```python
from build123d import *

# Parameters (mm, degrees)
F0_R     = 69.85
F1_DEPTH = 76.2
F2_DEPTH = 50.8
F3_DEPTH = 63.5
F4_DEPTH = 25.4


with BuildPart() as f1:
    # F0 (on Top) → F1 (new body)
    with BuildSketch(Plane.XY):
        Circle(F0_R)
        with BuildLine():
            ThreePointArc((33.3375, 57.7422437973), (52.8968339639, 40.5891682792), (64.4031044678, 17.2567598322))
            ThreePointArc((64.4031044678, 17.2567598322), (66.1045861321, 8.7028338663), (66.675, 0))
            ThreePointArc((66.675, 0), (66.1045861321, -8.7028338663), (64.4031044678, -17.2567598322))
            ThreePointArc((64.4031044678, -17.2567598322), (40.5891682792, -52.8968339639), (0, -66.675))
            ThreePointArc((0, -66.675), (-17.2567598322, -64.4031044678), (-33.3375, -57.7422437973))
            ThreePointArc((-33.3375, -57.7422437973), (-52.8968339639, -40.5891682792), (-64.4031044678, -17.2567598322))
            ThreePointArc((-64.4031044678, -17.2567598322), (-66.675, 0), (-64.4031044678, 17.2567598322))
            ThreePointArc((-64.4031044678, 17.2567598322), (-40.5891682792, 52.8968339639), (0, 66.675))
            ThreePointArc((0, 66.675), (17.2567598322, 64.4031044678), (33.3375, 57.7422437973))
        make_face(mode=Mode.SUBTRACT)
        with BuildLine():
            Line((-33.3375, -57.7422437973), (-31.75, -54.9926131403))
            ThreePointArc((-31.75, -54.9926131403), (-50.3779371085, -38.6563507421), (-61.3362899694, -16.435009364))
            Line((-61.3362899694, -16.435009364), (-64.4031044678, -17.2567598322))
            ThreePointArc((-64.4031044678, -17.2567598322), (-52.8968339639, -40.5891682792), (-33.3375, -57.7422437973))
        make_face()
        with BuildLine():
            ThreePointArc((-61.3362899694, 16.435009364), (-38.6563507421, 50.3779371085), (0, 63.5))
            Line((0, 63.5), (0, 66.675))
            ThreePointArc((0, 66.675), (-40.5891682792, 52.8968339639), (-64.4031044678, 17.2567598322))
            Line((-64.4031044678, 17.2567598322), (-61.3362899694, 16.435009364))
        make_face()
        with BuildLine():
            ThreePointArc((-61.3362899694, -16.435009364), (-63.5, 0), (-61.3362899694, 16.435009364))
            Line((-61.3362899694, 16.435009364), (-64.4031044678, 17.2567598322))
            ThreePointArc((-64.4031044678, 17.2567598322), (-66.675, 0), (-64.4031044678, -17.2567598322))
            Line((-64.4031044678, -17.2567598322), (-61.3362899694, -16.435009364))
        make_face()
        with BuildLine():
            ThreePointArc((61.3362899694, 16.435009364), (62.9567486972, 8.288413206), (63.5, 0))
            ThreePointArc((63.5, 0), (62.9567486972, -8.288413206), (61.3362899694, -16.435009364))
            Line((61.3362899694, -16.435009364), (64.4031044678, -17.2567598322))
            ThreePointArc((64.4031044678, -17.2567598322), (66.1045861321, -8.7028338663), (66.675, 0))
            ThreePointArc((66.675, 0), (66.1045861321, 8.7028338663), (64.4031044678, 17.2567598322))
            Line((64.4031044678, 17.2567598322), (61.3362899694, 16.435009364))
        make_face()
        with BuildLine():
            ThreePointArc((31.75, 54.9926131403), (50.3779371085, 38.6563507421), (61.3362899694, 16.435009364))
            Line((61.3362899694, 16.435009364), (64.4031044678, 17.2567598322))
            ThreePointArc((64.4031044678, 17.2567598322), (52.8968339639, 40.5891682792), (33.3375, 57.7422437973))
            Line((33.3375, 57.7422437973), (31.75, 54.9926131403))
        make_face()
        with BuildLine():
            Line((64.4031044678, -17.2567598322), (61.3362899694, -16.435009364))
            ThreePointArc((61.3362899694, -16.435009364), (38.6563507421, -50.3779371085), (0, -63.5))
            Line((0, -63.5), (0, -66.675))
            ThreePointArc((0, -66.675), (40.5891682792, -52.8968339639), (64.4031044678, -17.2567598322))
        make_face()
        with BuildLine():
            Line((0, -66.675), (0, -63.5))
            ThreePointArc((0, -63.5), (-16.435009364, -61.3362899694), (-31.75, -54.9926131403))
            Line((-31.75, -54.9926131403), (-33.3375, -57.7422437973))
            ThreePointArc((-33.3375, -57.7422437973), (-17.2567598322, -64.4031044678), (0, -66.675))
        make_face()
        with BuildLine():
            ThreePointArc((0, 63.5), (16.435009364, 61.3362899694), (31.75, 54.9926131403))
            Line((31.75, 54.9926131403), (33.3375, 57.7422437973))
            ThreePointArc((33.3375, 57.7422437973), (17.2567598322, 64.4031044678), (0, 66.675))
            Line((0, 66.675), (0, 63.5))
        make_face()
    extrude(amount=F1_DEPTH)

    # F0 (on Top) → F2 (cut)
    with BuildSketch(Plane.XY):
        with BuildLine():
            ThreePointArc((-61.3362899694, -16.435009364), (-63.5, 0), (-61.3362899694, 16.435009364))
            Line((-61.3362899694, 16.435009364), (-64.4031044678, 17.2567598322))
            ThreePointArc((-64.4031044678, 17.2567598322), (-66.675, 0), (-64.4031044678, -17.2567598322))
            Line((-64.4031044678, -17.2567598322), (-61.3362899694, -16.435009364))
        make_face()
        with BuildLine():
            ThreePointArc((61.3362899694, 16.435009364), (62.9567486972, 8.288413206), (63.5, 0))
            ThreePointArc((63.5, 0), (62.9567486972, -8.288413206), (61.3362899694, -16.435009364))
            Line((61.3362899694, -16.435009364), (64.4031044678, -17.2567598322))
            ThreePointArc((64.4031044678, -17.2567598322), (66.1045861321, -8.7028338663), (66.675, 0))
            ThreePointArc((66.675, 0), (66.1045861321, 8.7028338663), (64.4031044678, 17.2567598322))
            Line((64.4031044678, 17.2567598322), (61.3362899694, 16.435009364))
        make_face()
        with BuildLine():
            Line((-33.3375, -57.7422437973), (-31.75, -54.9926131403))
            ThreePointArc((-31.75, -54.9926131403), (-50.3779371085, -38.6563507421), (-61.3362899694, -16.435009364))
            Line((-61.3362899694, -16.435009364), (-64.4031044678, -17.2567598322))
            ThreePointArc((-64.4031044678, -17.2567598322), (-52.8968339639, -40.5891682792), (-33.3375, -57.7422437973))
        make_face()
        with BuildLine():
            ThreePointArc((31.75, 54.9926131403), (50.3779371085, 38.6563507421), (61.3362899694, 16.435009364))
            Line((61.3362899694, 16.435009364), (64.4031044678, 17.2567598322))
            ThreePointArc((64.4031044678, 17.2567598322), (52.8968339639, 40.5891682792), (33.3375, 57.7422437973))
            Line((33.3375, 57.7422437973), (31.75, 54.9926131403))
        make_face()
    extrude(amount=F2_DEPTH, mode=Mode.SUBTRACT)

    # F0 (on Top) → F3 (cut)
    with BuildSketch(Plane.XY):
        with BuildLine():
            Line((0, -66.675), (0, -63.5))
            ThreePointArc((0, -63.5), (-16.435009364, -61.3362899694), (-31.75, -54.9926131403))
            Line((-31.75, -54.9926131403), (-33.3375, -57.7422437973))
            ThreePointArc((-33.3375, -57.7422437973), (-17.2567598322, -64.4031044678), (0, -66.675))
        make_face()
        with BuildLine():
            ThreePointArc((0, 63.5), (16.435009364, 61.3362899694), (31.75, 54.9926131403))
            Line((31.75, 54.9926131403), (33.3375, 57.7422437973))
            ThreePointArc((33.3375, 57.7422437973), (17.2567598322, 64.4031044678), (0, 66.675))
            Line((0, 66.675), (0, 63.5))
        make_face()
    extrude(amount=F3_DEPTH, mode=Mode.SUBTRACT)

    # F0 (on Top) → F4 (join)
    with BuildSketch(Plane.XY):
        with BuildLine():
            Line((-33.3375, -57.7422437973), (-31.75, -54.9926131403))
            ThreePointArc((-31.75, -54.9926131403), (-50.3779371085, -38.6563507421), (-61.3362899694, -16.435009364))
            Line((-61.3362899694, -16.435009364), (-64.4031044678, -17.2567598322))
            ThreePointArc((-64.4031044678, -17.2567598322), (-52.8968339639, -40.5891682792), (-33.3375, -57.7422437973))
        make_face()
        with BuildLine():
            Line((0, -66.675), (0, -63.5))
            ThreePointArc((0, -63.5), (-16.435009364, -61.3362899694), (-31.75, -54.9926131403))
            Line((-31.75, -54.9926131403), (-33.3375, -57.7422437973))
            ThreePointArc((-33.3375, -57.7422437973), (-17.2567598322, -64.4031044678), (0, -66.675))
        make_face()
        with BuildLine():
            ThreePointArc((31.75, 54.9926131403), (50.3779371085, 38.6563507421), (61.3362899694, 16.435009364))
            Line((61.3362899694, 16.435009364), (64.4031044678, 17.2567598322))
            ThreePointArc((64.4031044678, 17.2567598322), (52.8968339639, 40.5891682792), (33.3375, 57.7422437973))
            Line((33.3375, 57.7422437973), (31.75, 54.9926131403))
        make_face()
        with BuildLine():
            ThreePointArc((0, 63.5), (16.435009364, 61.3362899694), (31.75, 54.9926131403))
            Line((31.75, 54.9926131403), (33.3375, 57.7422437973))
            ThreePointArc((33.3375, 57.7422437973), (17.2567598322, 64.4031044678), (0, 66.675))
            Line((0, 66.675), (0, 63.5))
        make_face()
    extrude(amount=F4_DEPTH)


solid = f1.part
```
For this review, take the finished solid that the model builds, in its own axes (mm). A direction names the side the tool comes from. Coordinates: 2 decimals unless noted, no trailing zeros. Write each loop counter-clockwise with the first axis right and the second up, starting at its lowest first coordinate (ties: lowest second). Pieces come first, ordered by that corner, then holes. Notation, with made-up numbers: (72.5, 45) - (92.5, 45) arc R32 ccw to (92.5, 71) - close; hole circle Ø11 at (2, 74.25). An arc over 180 degrees is marked (long way). Put each result on its own line as item: value.
1. Machinability: for faces 1 (the flat face through (15, -62, 76.2)), 2 (the flat face through (59.5, 23.2, 50.8)), which of the approach directions +Z, -Z, +X, -X, +Y, -Y give a long, thin tool a straight path to every point of the face, cutting with its end or side? Answer none if there is none.
Values found:
face 1: +Z, +X, -X, +Y, -Y
face 2: none
2. For pin 1 (1 mm diameter, centred on y = -16.5, z = 31.5, fed in from -X); pin 2 (6 mm diameter, centred on y = -10, z = 58.5, fed in from -X); pin 3 (3 mm diameter, centred on y = -38, z = 12, fed in from +X); pin 4 (12 mm diameter, centred on x = -42, y = -34, fed in from +Z), all flat-tipped, find the tip position at first contact; note any pin that passes through.
Values found:
pin 1: x = -67.99
pin 2: x = -69.5
pin 3: x = 59.55
pin 4: through
3. Add section A-A, the plane z = 13. Give the boundary of the cut face in (x, y) (3 decimals), then the cut area to 3 significant figures.
Values found:
outline: circle Ø139.7 at (0, 0); hole (-64.403, -17.257) - (-61.336, -16.435) arc R63.5 ccw to (61.336, -16.435) - (64.403, -17.257) arc R66.675 ccw to (64.403, 17.257) - (61.336, 16.435) arc R63.5 ccw to (-61.336, 16.435) - (-64.403, 17.257) arc R66.675 ccw to start
area: 2,440 mm²
4. Wall thickness on probe 1 along X at (y, z) = (39, 42); probe 2 along X at (y, z) = (49.5, 16); probe 3 along Y at (x, z) = (27.5, 40.5): over which ranges is each line inside the solid? List them lowest first.
Values found:
probe 1: -57.95 to -50.11, 54.08 to 57.95
probe 2: -49.28 to -39.77, 39.77 to 49.28
probe 3: -64.21 to -57.24, 60.74 to 64.21
5. Mouldability with a two-part tool opening along Y and no side actions: class faces 3 (the flat face through (15, -62, 0)), 4 (the cylindrical face through (-55.431, -42.503, 37.567)), 5 (the flat face through (-40, -51, 25.4)) as released by +Y, released by -Y, zero draft, split by the parting line, or undercut.
Values found:
face 3: zero draft
face 4: split by the parting line
face 5: undercut
6. Add section B-B, the plane x = -22. Give the boundary of the cut face in (y, z), then the cut area to 3 significant figures.
Values found:
outline: (-66.29, 0) - (-59.57, 0) - (-59.57, 25.4) - (-62.94, 25.4) - (-62.94, 63.5) - (-59.57, 63.5) - (-59.57, 76.2) - (-66.29, 76.2) - close; (59.57, 0) - (66.29, 0) - (66.29, 76.2) - (59.57, 76.2) - close
area: 897 mm²
7. Add section D-D, the plane x = 4.5. Give the boundary of the cut face in (y, z), then the cut area to 3 significant figures.
Values found:
outline: (-69.7, 0) - (-63.34, 0) - (-63.34, 76.2) - (-69.7, 76.2) - close; (63.34, 0) - (69.7, 0) - (69.7, 76.2) - (63.34, 76.2) - (63.34, 63.5) - (66.52, 63.5) - (66.52, 25.4) - (63.34, 25.4) - close
area: 849 mm²
